Input: dimensioned drawing with shaded views. Units: mm. Origin: part minimum x, y, z. A direction names the side the tool comes from. Coordinates: 2 decimals unless noted, no trailing zeros. Loops run counter-clockwise (first coordinate to the right, second up) from the corner with the lowest first, then second, coordinate; pieces in that order, holes last. Notation, with made-up numbers: (-34, 4.25) - (25, 4.25) arc R20 cw to (25, 19.25) - close; hole circle Ø3 at (27.5, 62.5). An arc over 180 degrees is marked (long way). Put each result on its own line as item: value. Start each with the question number.
1) Section A-A on z = 3.75. Output: boundary loops of the cut face in (x, y) (1 decimal).
2) Draft query along Y for the marked faces 1, 2, 3 and 4. Return one class per face: +Y half, -Y half, draft (parallel to the pull), parting line (faces both ways), or undercut.
3) Section D-D on y = 34.5. Output: boundary loops of the cut face in (x, z), and give its area (3 significant figures).
4) Contact query for flat-ended pins moving along their axis: pin 1 Ø3 at (y, z) = (33.5, 8.5) entering from -X; pin 2 Ø5 at (x, z) = (23.5, 7.5) entering from -Y. Output: stop coordinate, or through.
5) Section B-B on y = 25.36. Output: boundary loops of the cut face in (x, z).
6) Material intervals for line 1 along X through (y, z) = (49.5, 9); line 2 along Y through (x, z) = (37.5, 5.5); line 3 along Y through (x, z) = (21.5, 8.5) (1 decimal), sorted ascending. Write a range as from..to.
7) Section C-C on x = 22. Output: boundary loops of the cut face in (y, z).
8) Reachability of the marked faces 5 and 6 from +Z, -Z, +X, -X, +Y, -Y: full face, straight path, thin tool, end or side. Return the list, or none.
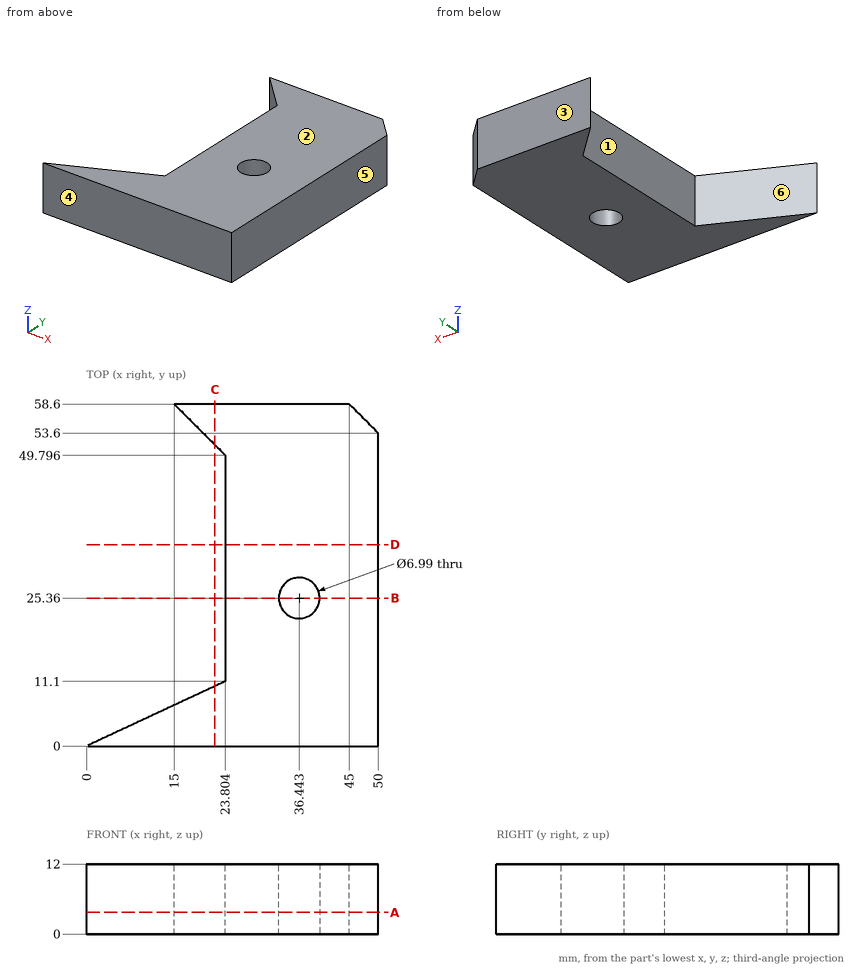
Answer block:
1. outline: (0, 0) - (50, 0) - (50, 53.6) - (45, 58.6) - (15, 58.6) - (23.8, 49.8) - (23.8, 11.1) - close; hole circle Ø7 at (36.4, 25.4)
2. face 1: undercut
2. face 2: draft
2. face 3: +Y half
2. face 4: -Y half
3. outline: (23.8, 0) - (50, 0) - (50, 12) - (23.8, 12) - close
3. area: 314 mm²
4. pin 1: stops at x = 23.8
4. pin 2: stops at y = 0
5. outline: (23.8, 0) - (32.95, 0) - (32.95, 12) - (23.8, 12) - close; (39.94, 0) - (50, 0) - (50, 12) - (39.94, 12) - close
6. line 1: x = 23.8..50
6. line 2: y = 0..22.03, 28.69..58.6
6. line 3: y = 0..10, 52.1..58.6
7. outline: (0, 0) - (10.26, 0) - (10.26, 12) - (0, 12) - close; (51.6, 0) - (58.6, 0) - (58.6, 12) - (51.6, 12) - close
8. face 5: +Z, -Z, +X, +Y, -Y
8. face 6: +Z, -Z, -X
